from build123d import *


with BuildPart() as f1:
    # F0 (on Front) → F1 (revolve)
    with BuildSketch(Plane.XZ):
        with BuildLine():
            ThreePointArc((0, 14.736695), (-0.01711, 14.997747), (-0.068148, 15.254333))
            Line((-0.068148, 15.254333), (-3.338541, 27.459603))
            ThreePointArc((-3.338541, 27.459603), (-3.538341, 27.941965), (-3.856179, 28.356179))
            Line((-3.856179, 28.356179), (-4.914214, 29.414214))
            ThreePointArc((-4.914214, 29.414214), (-5.56306, 29.847759), (-6.328427, 30))
            Line((-6.328427, 30), (-8, 30))
            Line((-8, 30), (-10, 28))
            Line((-10, 28), (-12, 30))
            Line((-12, 30), (-13, 30))
            ThreePointArc((-13, 30), (-14.4142, 29.414227), (-15, 28.000038))
            Line((-15, 28.000038), (-15, 0))
            Line((-15, 0), (-10, 0))
            Line((-10, 0), (-10, 3.3))
            Line((-10, 3.3), (-2.8, 3.3))
            Line((-2.8, 3.3), (-2.8, 5.1))
            Line((-2.8, 5.1), (0, 5.1))
            Line((0, 5.1), (0, 14.736695))
        make_face()
    revolve(axis=Axis((-0.70766, 0, 0), (1, 0, 0)))


solid = f1.part
Work out the finished part from the listing and answer in its coordinate system (mm). A direction names the side the tool comes from. Round coordinates to 2 decimals unless told otherwise and drop trailing zeros. Write each question's results on one line, items separated by ' | '.
Item 1: The mould has two halves that part along X. Classify faces 3 (the face through (-10, 0, 0)), 4 (the face through (-10.13, -8.45, 26.83)), 5 (the face through (-6.35, -2.23, -2.43)): +X half, -X half, draft (parallel to the pull), parting line (faces both ways), or undercut.
Result set:
face 3: +X half | face 4: undercut | face 5: draft
Item 2: Find the intervals of material crossed by line 1 along Z through (x, y) = (-7, 0); line 2 along Y through (x, z) = (-4.5, 0); line 3 along Z through (x, y) = (-8.25, 0), in increasing order. Write a range as [from, to].
Result set:
line 1: [-30, -3.3], [3.3, 30] | line 2: [-29, -3.3], [3.3, 29] | line 3: [-29.75, -3.3], [3.3, 29.75]
Item 3: Which of the six approach directions +Z, -Z, +X, -X, +Y, -Y give full straight-line access (tool end or side, diameter ignored) to faces 1 (the face through (-7.18, -1.32, -29.97)), 2 (the face through (-2.8, 1.1, -3.3))?
Result set:
face 1: +X, -X | face 2: +X
Item 4: Flat-ended cylindrical pins translate along their axes: P1, Ø7.5, axis at y = 1, z = 0, coming from the +X side; P2, Ø3, axis at y = 0.5, z = -1.5, coming from the +X side; P3, Ø4, axis at x = -8, y = -12, coming from the -Z side. Find the tip coordinate at first contact, or state that the pin passes through.
Result set:
P1: x = -2.8 | P2: x = -10 | P3: z = -28.28
